Build history of the part. All positions in model axes, mm. Give positions to 0.01 mm unless a question says otherwise; leave off trailing zeros. Write each loop counter-clockwise with the first axis right and the second up, starting at its lowest first coordinate (ties: lowest second). Pieces come first, ordered by that corner, then holes. Notation, with made-up numbers: (24.5, -21) -> (75.5, -21) arc R36 ccw to (75.5, 18) -> close; hole circle Ø10 at (71, 13). An arc over 180 degrees is marked (long way). Put each result on its own line as item: value.
from build123d import *

# Parameters (mm, degrees)
SKETCH1_W           = 3
SKETCH1_H           = 10
SKETCH1_W_2         = 10
SKETCH1_H_2         = 3
BOSS_EXTRUDE1_DEPTH = 2.5
SKETCH2_W           = 10
SKETCH2_H           = 3
CUT_EXTRUDE1_DEPTH  = 10
SKETCH3_R           = 5
SKETCH3_W           = 25
SKETCH3_H           = 10
CUT_EXTRUDE2_DEPTH  = 10


with BuildPart() as part:
    # Sketch1 → Boss-Extrude1 (new body)
    with BuildSketch(Plane(origin=(0, 0, 0), x_dir=(1, 0, 0), z_dir=(0, 1, 0))):
        Polygon((0, 0), (0, 50), (-3, 50), (-3, 80), (0, 80), (0, 210), (-3, 210), (-3, 240), (0, 240), (0, 370), (-3, 370), (-3, 400), (0, 400), (0, 450), (30, 450), (30, 453), (60, 453), (60, 450), (160, 450), (160, 453), (190, 453), (190, 450), (220, 450), (220, 400), (223, 400), (223, 370), (220, 370), (220, 250), (223, 250), (223, 220), (220, 220), (220, 100), (223, 100), (223, 70), (220, 70), (220, 40), (270, 40), (270, 43), (300, 43), (300, 40), (360, 40), (360, 43), (390, 43), (390, 40), (450, 40), (450, 43), (480, 43), (480, 40), (530, 40), (530, 70), (527, 70), (527, 100), (530, 100), (530, 180), (527, 180), (527, 210), (530, 210), (530, 290), (527, 290), (527, 320), (530, 320), (530, 350), (555, 350), (555, 353), (585, 353), (585, 350), (610, 350), (610, 320), (613, 320), (613, 290), (610, 290), (610, 210), (613, 210), (613, 180), (610, 180), (610, 100), (613, 100), (613, 70), (610, 70), (610, 0), (560, 0), (560, -3), (530, -3), (530, 0), (400, 0), (400, -3), (370, -3), (370, 0), (240, 0), (240, -3), (210, -3), (210, 0), (80, 0), (80, -3), (50, -3), (50, 0), align=None)
        with Locations((68.5, 265)):
            Rectangle(SKETCH1_W, SKETCH1_H, mode=Mode.SUBTRACT)
        with Locations((68.5, 285)):
            Rectangle(SKETCH1_W, SKETCH1_H, mode=Mode.SUBTRACT)
        with Locations((85, 258.5)):
            Rectangle(SKETCH1_W_2, SKETCH1_H_2, mode=Mode.SUBTRACT)
        with Locations((135, 258.5)):
            Rectangle(SKETCH1_W_2, SKETCH1_H_2, mode=Mode.SUBTRACT)
        with Locations((151.5, 265)):
            Rectangle(SKETCH1_W, SKETCH1_H, mode=Mode.SUBTRACT)
        with Locations((151.5, 285)):
            Rectangle(SKETCH1_W, SKETCH1_H, mode=Mode.SUBTRACT)
    extrude(amount=BOSS_EXTRUDE1_DEPTH)

    # Sketch2 → Cut-Extrude1 (cut)
    with BuildSketch(Plane(origin=(0, 2.5, 0), x_dir=(1, 0, 0), z_dir=(0, 1, 0))):
        with Locations((537.5, 272.5)):
            Rectangle(SKETCH2_W, SKETCH2_H)
    extrude(amount=-CUT_EXTRUDE1_DEPTH, mode=Mode.SUBTRACT)

    # Sketch3 → Cut-Extrude2 (cut)
    with BuildSketch(Plane.XZ):
        with Locations(Location((25, -25, 0), (0, 0, 270))):
            Circle(SKETCH3_R)
        with Locations((87.5, -270)):
            Rectangle(SKETCH3_W, SKETCH3_H)
    extrude(amount=-CUT_EXTRUDE2_DEPTH, mode=Mode.SUBTRACT)


solid = part.part
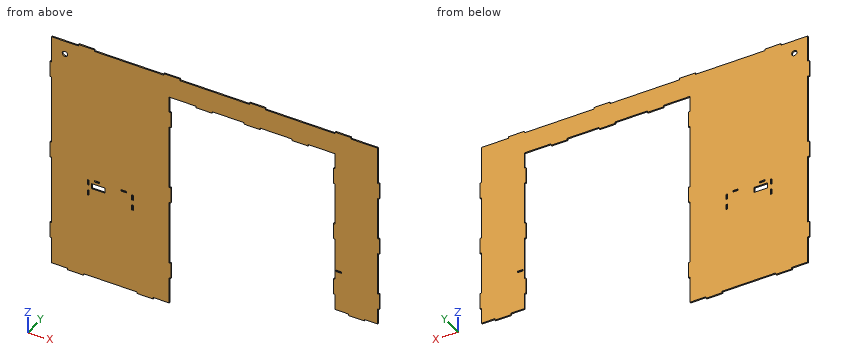
1) Wall check: L1, parallel to X at y = 0.9, z = -286.5; L2, parallel to Z at x = 221, y = 1.55; L3, parallel to X at y = 1.05, z = -322. Give the ranges that are in metal, low to high.
Filled sheet:
L1: 0 to 67, 70 to 150, 153 to 220, 530 to 610
L2: -400 to -370, -250 to -220, -100 to -70, -40 to 3
L3: 0 to 220, 530 to 610
2) Slice it at B-B (y = 2). Give the number of separate pieces and of enclosed holes in the cut face, plus the area to 3 significant figures.
Filled sheet:
separate pieces: 1
enclosed holes: 9
area: 141,000 mm2
3) Slice it at A-A (z = -108). Write the cut outline in (x, y), plus the area to 3 significant figures.
Filled sheet:
outline: (0, 0) -> (220, 0) -> (220, 2.5) -> (0, 2.5) -> close; (530, 0) -> (610, 0) -> (610, 2.5) -> (530, 2.5) -> close
area: 750 mm2
4) Pin check, flat tips, straight feed: pin 1 (1.2 mm diameter, centred on x = 151.5, y = 1, fed in from +Z); pin 2 (1.2 mm diameter, centred on y = 1.5, z = -41.5, fed in from +X); pin 3 (0.8 mm diameter, centred on x = 538, y = 1, fed in from -Z). Stop position of each tip, or through.
Filled sheet:
pin 1: z = 0
pin 2: x = 610
pin 3: z = -350
